from build123d import *

# Parameters (mm, degrees)
SKETCH_1_R          = 2.5
EXTRUDE_1_DEPTH     = 72
CUT_EXTRUDE_START   = -15
CUT_EXTRUDE_1_DEPTH = 15
CHAMFER_1_SIZE      = 0.5


with BuildPart() as part:
    # Эскиз1 → Бобышка-Вытянуть1 (new body)
    with BuildSketch(Plane(origin=(0, 0, 0), x_dir=(1, 0, 0), z_dir=(0, 1, 0))):
        with Locations(Location((0, 0, 0), (0, 0, 270))):
            Circle(SKETCH_1_R)
    extrude(amount=EXTRUDE_1_DEPTH)

    # Эскиз2 → Вырез-Вытянуть1 (cut)
    with BuildSketch(Plane(origin=(0, 72, 0), x_dir=(1, 0, 0), z_dir=(0, 1, 0)).offset(CUT_EXTRUDE_START)):
        with BuildLine():
            Line((-1.5, 2), (1.5, 2))
            ThreePointArc((1.5, 2), (0, 2.5), (-1.5, 2))
        make_face()
    extrude(amount=CUT_EXTRUDE_1_DEPTH, mode=Mode.SUBTRACT)

    # Фаска1
    chamfer_1_edges = [part.edges().sort_by_distance(p)[0] for p in [
        (-2.371708245, 72, 0.790569415),
        (0, 0, -2.5),
    ]]
    chamfer(chamfer_1_edges, length=CHAMFER_1_SIZE - 0.0001)  # a hair under: the kernel refuses the full size


solid = part.part
Build history of the part. All positions in model axes, mm. A direction names the side the tool comes from. Round coordinates to 2 decimals unless told otherwise and drop trailing zeros. Write each loop counter-clockwise with the first axis right and the second up, starting at its lowest first coordinate (ties: lowest second). Pieces come first, ordered by that corner, then holes. Notation, with made-up numbers: M 89,84 L 124,84 A9 ccw 124,91 Z; hole C -30,39.25 d5. An arc over 180 degrees is marked long. Use CSV: the item, a comma, the result in double quotes.
1. Saw through at A-A (y = 38). Give the cut face in (x, z).
Reply:
outline,"C 0,0 d5"
2. Wall check: probe 1 along X at (y, z) = (50.5, -1.5); probe 2 along X at (y, z) = (55.5, -0.45); probe 3 along Z at (x, y) = (0.6, 58). Give the ranges that are in metal, low to high. Write a range as from..to.
Reply:
probe 1,"x = -2..2"
probe 2,"x = -2.46..2.46"
probe 3,"z = -2..2.43"
3. Tool access for faces 1 (the face through (0.751, 35.503, 2.385)), 2 (the face through (0, 64, -2)): list every direction of +Z, -Z, +X, -X, +Y, -Y with a clear straight run to the whole face (end or side of a thin tool).
Reply:
face 1,"+Y, -Y"
face 2,"-Z, +X, -X, +Y"
4. Saw through at B-B (y = 61.5). Give the cut face in (x, z), plus the area to 3 significant figures.
Reply:
outline,"M -1.5,-2 L 1.5,-2 A2.5 ccw long Z"
area,"18.6 mm²"
